```python
from build123d import *

# Parameters (mm, degrees)
F0_W      = 40
F0_H      = 5
F1_DEPTH  = 120
F2_W      = 20
F2_H      = 5
F3_DEPTH  = 120
F4_W      = 120
F4_H      = 40
F5_DEPTH  = 5
F6_W      = 40
F6_H      = 5
F7_DEPTH  = 35
F8_W      = 40
F8_H      = 5
F9_DEPTH  = 35
F10_W     = 40
F10_H     = 5
F11_DEPTH = 35
F12_W     = 40
F12_H     = 5
F13_DEPTH = 35


with BuildPart() as f1:
    # F0 (on Right) → F1 (new body)
    with BuildSketch(Plane.YZ):
        with Locations((-7.7903409343, -32.0171793364)):
            Rectangle(F0_W, F0_H)
    extrude(amount=F1_DEPTH)

    # F2 (on face) → F3 (join)
    with BuildSketch(Plane.XY.offset(-29.5171793364)):
        Polygon((45, 12.2096590657), (40, 12.2096590657), (40, -27.7903409343), (60, -27.7903409343), (60, -22.7903409343), (45, -22.7903409343), align=None)
        with Locations((70, -25.2903409343)):
            Rectangle(F2_W, F2_H)
    extrude(amount=F3_DEPTH)

    # F4 (on face) → F5 (join)
    with BuildSketch(Plane.XY.offset(90.4828206636)):
        with Locations((60, -7.7903409343)):
            Rectangle(F4_W, F4_H)
    extrude(amount=F5_DEPTH)

    # F6 (on face) → F7 (join)
    with BuildSketch(Plane.XY.offset(-29.5171793364)):
        with Locations((20, -25.2903409343)):
            Rectangle(F6_W, F6_H)
    extrude(amount=F7_DEPTH)

    # F8 (on face) → F9 (join)
    with BuildSketch(Plane.XY.offset(-29.5171793364)):
        with Locations((100, -25.2903409343)):
            Rectangle(F8_W, F8_H)
    extrude(amount=F9_DEPTH)

    # F10 (on face) → F11 (join)
    with BuildSketch(Plane(origin=(0, 0, 90.4828206636), x_dir=(1, 0, 0), z_dir=(0, 0, -1))):
        with Locations((20, 25.2903409343)):
            Rectangle(F10_W, F10_H)
    extrude(amount=F11_DEPTH)

    # F12 (on face) → F13 (join)
    with BuildSketch(Plane(origin=(0, 0, 90.4828206636), x_dir=(1, 0, 0), z_dir=(0, 0, -1))):
        with Locations((100, 25.2903409343)):
            Rectangle(F12_W, F12_H)
    extrude(amount=F13_DEPTH)


solid = f1.part
```
Could you check a few things on this model? Use its own coordinates, in mm. A direction names the side the tool comes from. Coordinates: 2 decimals unless noted, no trailing zeros. Write each loop counter-clockwise with the first axis right and the second up, starting at its lowest first coordinate (ties: lowest second). Pieces come first, ordered by that corner, then holes. Notation, with made-up numbers: M -11.75,81.25 L 18.25,81.25 A8 cw 18.25,96.25 Z; hole C -34.5,58 d6. An arc over 180 degrees is marked long. Answer as CSV lines item,"result". Start each with the question number.
1) I want a section at D-D, the plane z = 67.5. Please give me the cut outline in (x, y).
2) I want a section at A-A, the plane x = 85. Please give me the cut outline in (y, z), and give its area (3 significant figures).
3) I want a section at B-B, the plane y = -14.5. Please give me the cut outline in (x, z), and give its area (3 significant figures).
4) We'd pull the mould along Z, two halves only. Please class faces 4 (the flat face through (45, -6, 30)), 5 (the flat face through (0, -15, 92)), 6 (the flat face through (59, -8, -34.517)): +Z half, -Z half, draft (parallel to the pull), parting line (faces both ways), or undercut.
5) For faces 1 (the flat face through (100, -25, 55.483)), 2 (the flat face through (20, -22.79, 73)), 3 (the flat face through (82, -6, -29.517)), which set-ups out of +Z, -Z, +X, -X, +Y, -Y let a thin tool reach every point of the face, with its end or its side?
6) For P1, Ø20, axis at y = 0, z = 32, coming from the -X side; P2, Ø22.5, axis at x = 78, z = 55, coming from the +Y side; P3, Ø1.5, axis at y = -25, z = 42, coming from the +X side; P4, Ø5, axis at y = -22, z = 65.5, coming from the +X side, each with a flat end and sliding along its axis, tell me the tip position at first contact or that it passes through.
7) Please list where these lines run through material, in increasing order: line 1 (Z direction, x = 23, y = -1.5); line 2 (Y direction, x = 12, z = 71.5); line 3 (X direction, y = -26, z = 8). Write a range as from..to.
8) I want a section at C-C, the plane x = 47.5. Please give me the cut outline in (y, z).
Data:
1,outline,"M 0,-27.79 L 120,-27.79 L 120,-22.79 L 45,-22.79 L 45,12.21 L 40,12.21 L 40,-22.79 L 0,-22.79 Z"
2,outline,"M -27.79,-34.52 L 12.21,-34.52 L 12.21,-29.52 L -22.79,-29.52 L -22.79,5.48 L -27.79,5.48 Z; M -27.79,55.48 L -22.79,55.48 L -22.79,90.48 L 12.21,90.48 L 12.21,95.48 L -27.79,95.48 Z"
2,area,"750 mm^2"
3,outline,"M 0,-34.52 L 120,-34.52 L 120,-29.52 L 45,-29.52 L 45,90.48 L 120,90.48 L 120,95.48 L 0,95.48 L 0,90.48 L 40,90.48 L 40,-29.52 L 0,-29.52 Z"
3,area,"1,800 mm^2"
4,face 4,"undercut"
4,face 5,"draft"
4,face 6,"-Z half"
5,face 1,"+X, +Y, -Y"
5,face 2,"-X, +Y"
5,face 3,"+X, +Y"
6,P1,"stops at x = 40"
6,P2,"stops at y = -22.79"
6,P3,"stops at x = 80"
6,P4,"stops at x = 120"
7,line 1,"z = -34.52..-29.52, 90.48..95.48"
7,line 2,"y = -27.79..-22.79"
7,line 3,"x = 40..80"
8,outline,"M -27.79,-34.52 L 12.21,-34.52 L 12.21,-29.52 L -22.79,-29.52 L -22.79,90.48 L 12.21,90.48 L 12.21,95.48 L -27.79,95.48 Z"
